Source: CAD feature listing. Evaluate the final solid. Frame: model axes, mm. Give positions to 0.01 mm unless a question says otherwise; leave off trailing zeros. Order: outer loops, then holes, each group sorted by start corner. A loop starts at its lowest first (then second) coordinate and runs counter-clockwise, first axis right, second up.
```python
from build123d import *

# Parameters (mm, degrees)
SKETCH1_W                 = 50
SKETCH1_H                 = 6.35
BOSS_EXTRUDE1_DEPTH       = 25
M4X0_7_TAPPED_HOLE1_D     = 3.3
M4X0_7_TAPPED_HOLE1_DEPTH = 10.1
M4X0_7_TAPPED_HOLE1_TIP   = 0.991420021
M4X0_7_TAPPED_HOLE2_D     = 3.3
M4X0_7_TAPPED_HOLE2_DEPTH = 10.1
M4X0_7_TAPPED_HOLE2_TIP   = 0.991420021


with BuildPart() as part:
    # Sketch1 → Boss-Extrude1 (new body)
    with BuildSketch(Plane(origin=(0, 0, 0), x_dir=(1, 0, 0), z_dir=(0, 1, 0))):
        with Locations((25, 3.175)):
            Rectangle(SKETCH1_W, SKETCH1_H)
    extrude(amount=BOSS_EXTRUDE1_DEPTH)

    # M4x0.7 Tapped Hole1
    with Locations(Plane(origin=(40, 25, -3.175), x_dir=(0, 0, 1), z_dir=(0, 1, 0))):
        with Locations((0, 0), (0, -30)):
            Hole(M4X0_7_TAPPED_HOLE1_D / 2, depth=M4X0_7_TAPPED_HOLE1_DEPTH)
            with Locations((0, 0, -(M4X0_7_TAPPED_HOLE1_DEPTH + M4X0_7_TAPPED_HOLE1_TIP / 2))):  # 118° drill point
                Cone(0, M4X0_7_TAPPED_HOLE1_D / 2, M4X0_7_TAPPED_HOLE1_TIP, mode=Mode.SUBTRACT)

    # M4x0.7 Tapped Hole2
    with Locations(Plane(origin=(5, 21.5, 0), x_dir=(1, 0, 0), z_dir=(0, 0, 1))):
        with Locations((0, 0), (40, 0), (40, -18), (0, -18)):
            Hole(M4X0_7_TAPPED_HOLE2_D / 2, depth=M4X0_7_TAPPED_HOLE2_DEPTH)
            with Locations((0, 0, -(M4X0_7_TAPPED_HOLE2_DEPTH + M4X0_7_TAPPED_HOLE2_TIP / 2))):  # 118° drill point
                Cone(0, M4X0_7_TAPPED_HOLE2_D / 2, M4X0_7_TAPPED_HOLE2_TIP, mode=Mode.SUBTRACT)


solid = part.part
```
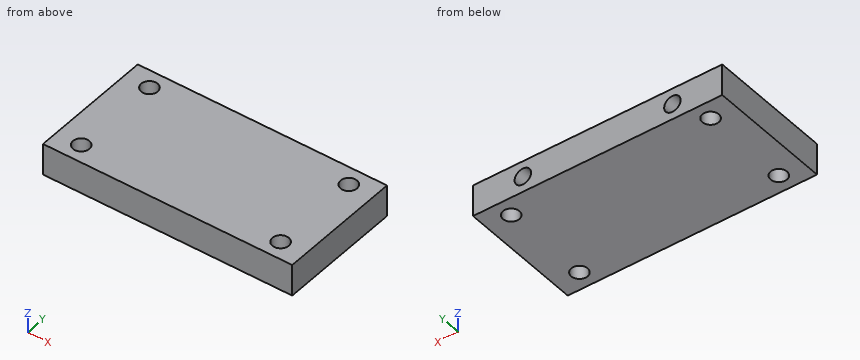
1) Material intervals for L1, parallel to Y at x = 45, z = -1.75; L2, parallel to X at y = 15.5, z = -3; L3, parallel to Z at x = 40, y = 21.25 (3 decimals), sorted ascending.
Report:
L1: y = 0 to 1.85, 5.15 to 19.85, 23.15 to 25
L2: x = 0 to 8.36, 11.64 to 38.36, 41.64 to 50
L3: z = -6.35 to -4.825, -1.525 to 0
2) Section query B-B, the plane z = -0.5. Return the cut outline in (x, y), and give its area (3 significant figures).
Report:
outline: (0, 0) - (50, 0) - (50, 25) - (0, 25) - close; hole circle Ø3.3 at (5, 3.5); hole circle Ø3.3 at (5, 21.5); hole circle Ø3.3 at (45, 3.5); hole circle Ø3.3 at (45, 21.5)
area: 1,220 mm2
3) Section query C-C, the plane y = 3.5. Return the cut outline in (x, z).
Report:
outline: (0, -6.35) - (3.35, -6.35) - (3.35, 0) - (0, 0) - close; (6.65, -6.35) - (43.35, -6.35) - (43.35, 0) - (6.65, 0) - close; (46.65, -6.35) - (50, -6.35) - (50, 0) - (46.65, 0) - close
4) Pin query (flat end, axial travel): pin 1 (2.5 mm diameter, centred on x = 45, y = 21.5, fed in from -Z). Return the tip coordinate at first contact, or that it passes through.
Report:
pin 1: passes through
5) Section query A-A, the plane y = 21.5. Return the cut outline in (x, z) (3 decimals), and give its area (3 significant figures).
Report:
outline: (0, -6.35) - (3.35, -6.35) - (3.35, 0) - (0, 0) - close; (6.65, -6.35) - (43.35, -6.35) - (43.35, 0) - (6.65, 0) - close; (46.65, -6.35) - (50, -6.35) - (50, 0) - (46.65, 0) - close; hole circle Ø3.3 at (10, -3.175); hole circle Ø3.3 at (40, -3.175)
area: 258 mm2
6) Section query D-D, the plane x = 45. Return the cut outline in (y, z).
Report:
outline: (0, -6.35) - (1.85, -6.35) - (1.85, 0) - (0, 0) - close; (5.15, -6.35) - (19.85, -6.35) - (19.85, 0) - (5.15, 0) - close; (23.15, -6.35) - (25, -6.35) - (25, 0) - (23.15, 0) - close
